Model file for the job. Use its own axes, mm. Face numbers are marked on the shaded views. A direction names the side the tool comes from. Coordinates: 2 decimals unless noted, no trailing zeros. Order: outer loops, then holes, each group sorted by start corner. A loop starts at its lowest first (then second) coordinate and runs counter-clockwise, first axis right, second up.
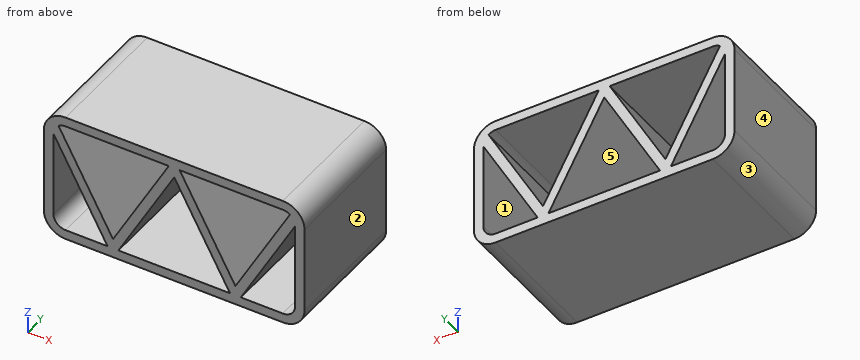
from build123d import *

# Parameters (mm, degrees)
EXTRUDE_THIN1_DEPTH = 304.8
EXTRUDE_THIN3_DEPTH = 304.8


with BuildPart() as part:
    # Sketch1 → Extrude-Thin1 (new body)
    with BuildSketch(Plane(origin=(0, 0, 0), x_dir=(1, 0, 0), z_dir=(0, 1, 0))):
        with BuildLine():
            Line((-254, 152.4), (254, 152.4))
            ThreePointArc((254, 152.4), (289.921024484, 137.521024484), (304.8, 101.6))
            Line((304.8, 101.6), (304.8, -101.6))
            ThreePointArc((304.8, -101.6), (289.921024484, -137.521024484), (254, -152.4))
            Line((254, -152.4), (-254, -152.4))
            ThreePointArc((-254, -152.4), (-289.921024484, -137.521024484), (-304.8, -101.6))
            Line((-304.8, -101.6), (-304.8, 101.6))
            ThreePointArc((-304.8, 101.6), (-289.921024484, 137.521024484), (-254, 152.4))
        make_face()
        with BuildLine():
            Line((-254, 130.175), (254, 130.175))
            ThreePointArc((254, 130.175), (274.205576272, 121.805576272), (282.575, 101.6))
            Line((282.575, 101.6), (282.575, -101.6))
            ThreePointArc((282.575, -101.6), (274.205576272, -121.805576272), (254, -130.175))
            Line((254, -130.175), (-254, -130.175))
            ThreePointArc((-254, -130.175), (-274.205576272, -121.805576272), (-282.575, -101.6))
            Line((-282.575, -101.6), (-282.575, 101.6))
            ThreePointArc((-282.575, 101.6), (-274.205576272, 121.805576272), (-254, 130.175))
        make_face(mode=Mode.SUBTRACT)
    extrude(amount=EXTRUDE_THIN1_DEPTH)

    # Sketch2 → Extrude-Thin3 (add)
    with BuildSketch(Plane(origin=(0, 304.8, 0), x_dir=(1, 0, 0), z_dir=(0, 1, 0))):
        with BuildLine():
            Line((-276.558924799, -135.529052432), (-143.148286149, 107.110665493))
            Line((-143.148286149, 107.110665493), (-11.963395498, -131.480987957))
            ThreePointArc((-11.963395498, -131.480987957), (0, -138.555652113), (11.963395498, -131.480987957))
            Line((11.963395498, -131.480987957), (143.148286149, 107.110665493))
            Line((143.148286149, 107.110665493), (276.558924799, -135.529052432))
            Line((276.558924799, -135.529052432), (296.034219796, -124.820947568))
            Line((296.034219796, -124.820947568), (155.111681647, 131.480987957))
            ThreePointArc((155.111681647, 131.480987957), (143.148286149, 138.555652113), (131.18489065, 131.480987957))
            Line((131.18489065, 131.480987957), (0, -107.110665493))
            Line((0, -107.110665493), (-131.18489065, 131.480987957))
            ThreePointArc((-131.18489065, 131.480987957), (-143.148286149, 138.555652113), (-155.111681647, 131.480987957))
            Line((-155.111681647, 131.480987957), (-296.034219796, -124.820947568))
            Line((-296.034219796, -124.820947568), (-276.558924799, -135.529052432))
        make_face()
    extrude(amount=-EXTRUDE_THIN3_DEPTH)


solid = part.part
Q1. Drop flat-ended pins along their axis: P1, Ø8, axis at y = 229, z = -119, coming from the +X side; P2, Ø5, axis at y = 261, z = -112, coming from the -X side. Give the stop position or say it passes through.
Established:
P1: stops at x = 303
P2: stops at x = -304.18
Q2. Mould opens along Z. For the marked faces 3, 4 and 5 say: pulls with the +Z half, pulls with the -Z half, needs draft (parallel to the pull), parting line crosses it, or undercut.
Established:
face 3: pulls with the -Z half
face 4: needs draft
face 5: undercut
Q3. Which spindle directions (+Z, -Z, +X, -X, +Y, -Y) get a long thin tool onto all of the face, cutting with end or side? Do the marked faces 1 and 2. Say none if no direction does.
Established:
face 1: +Y, -Y
face 2: +Z, -Z, +X, +Y, -Y
Q4. Cut at A-A, the plane y = 124. List the corners of the cut face in (x, z) (3 decimals).
Established:
outline: (-304.8, -101.6) arc R50.8 ccw to (-254, -152.4) - (254, -152.4) arc R50.8 ccw to (304.8, -101.6) - (304.8, 101.6) arc R50.8 ccw to (254, 152.4) - (-254, 152.4) arc R50.8 ccw to (-304.8, 101.6) - close; hole (-282.575, -101.6) arc R28.575 ccw to (-254, -130.175) - (-155.83, -130.175) - (-282.575, 100.342) - close; hole (-270.666, 124.811) - (-143.148, -107.111) - (-12.681, 130.175) - (-254, 130.175) arc R28.575 ccw to start; hole (-130.467, -130.175) - (130.467, -130.175) - (0, 107.111) - close; hole (12.681, 130.175) - (143.148, -107.111) - (270.666, 124.811) arc R28.575 ccw to (254, 130.175) - close; hole (155.83, -130.175) - (254, -130.175) arc R28.575 ccw to (282.575, -101.6) - (282.575, 100.342) - close
Q5. Cut at C-C, the plane z = -115. List the corners of the cut face in (x, y), plus the area to 3 significant figures.
Established:
outline: (-303, 0) - (-279.24, 0) - (-279.24, 304.8) - (-303, 304.8) - close; (-164.17, 0) - (-122.12, 0) - (-122.12, 304.8) - (-164.17, 304.8) - close; (122.12, 0) - (164.17, 0) - (164.17, 304.8) - (122.12, 304.8) - close; (279.24, 0) - (303, 0) - (303, 304.8) - (279.24, 304.8) - close
area: 40,100 mm2
Q6. Cut at B-B, the plane x = 264.5. List the corners of the cut face in (y, z).
Established:
outline: (0, -151.3) - (304.8, -151.3) - (304.8, -128.18) - (0, -128.18) - close; (0, 67.47) - (304.8, 67.47) - (304.8, 113.6) - (0, 113.6) - close; (0, 128.18) - (304.8, 128.18) - (304.8, 151.3) - (0, 151.3) - close
Q7. Probe line 1 (X direction, y = 256.5, z = 122.5); line 2 (Z direction, x = -215, y = 285) (1 decimal); line 3 (Z direction, x = -87.5, y = 289.5) (3 decimals). List the from-to ranges inside material, lowest first.
Established:
line 1: x = -300.3 to -269.4, -16.9 to 16.9, 269.4 to 300.3
line 2: z = -152.4 to -130.2, -22.6 to 23.6, 130.2 to 152.4
line 3: z = -152.4 to -130.175, -52.029 to -5.901, 130.175 to 152.4
Q8. Cut at D-D, the plane z = 10. List the corners of the cut face in (x, y) (3 decimals).
Established:
outline: (-304.8, 0) - (-282.575, 0) - (-282.575, 304.8) - (-304.8, 304.8) - close; (-232.902, 0) - (-207.539, 0) - (-207.539, 304.8) - (-232.902, 304.8) - close; (-78.757, 0) - (-53.394, 0) - (-53.394, 304.8) - (-78.757, 304.8) - close; (53.394, 0) - (78.757, 0) - (78.757, 304.8) - (53.394, 304.8) - close; (207.539, 0) - (232.902, 0) - (232.902, 304.8) - (207.539, 304.8) - close; (282.575, 0) - (304.8, 0) - (304.8, 304.8) - (282.575, 304.8) - close
